Input: part model. Units: mm. Frame: model coordinates. A direction names the side the tool comes from. Give positions to 0.01 mm unless a question says otherwise; leave off trailing zeros. Loops run counter-clockwise (first coordinate to the right, second up) from the corner with the lowest first, then second, coordinate; pieces in that order, holes last. Notation, with made-up numbers: M -27.75,-0.75 L 18.25,-0.75 A31 cw 18.25,36.25 Z; hole C 72.5,-33.75 d11. An arc over 180 degrees is marked long. Answer as a JSON object with one key per item and string values. Group by question number.
1) First-contact query: P1, Ø1.5, axis at y = 18, z = 618, coming from the -X side; P2, Ø6, axis at x = 7, y = 14.5, coming from the +Z side. Flat tips, straight axial feed; report the tip coordinate or a pass-through.
2) Ray query, L1, parallel to X at y = 7.75, z = 55.5 (3 decimals); L2, parallel to Y at x = 0.8, z = 12.7. Return the intervals inside material, ascending.
3) Access query for faces 1 (the flat face through (24, 13, 0)), 2 (the flat face through (13, 22.225, 376)). Directions: +Z, -Z, +X, -X, +Y, -Y. A direction counts if a zero-diameter tool reaches every point of the face in a straight line with its end or side. Return the directions, or none.
4) Section query C-C on y = 12.7. Return loops of the section in (x, z) (3 decimals).
5) Section query A-A on z = 12.7. Return loops of the section in (x, y) (3 decimals), plus the area to 3 significant figures.
6) Draft query along Y for faces 3 (the cylindrical face through (23.79, 16.99, 8.02)), 4 (the flat face through (13, 25.4, 376)), 5 (the flat face through (0, 13, 376)). Return one class per face: +Y half, -Y half, draft (parallel to the pull), parting line (faces both ways), or undercut.
7) Section query B-B on x = 10.5. Return loops of the section in (y, z) (3 decimals).
8) Section query D-D on z = 453.5. Return loops of the section in (x, y) (3 decimals).
Autodesk Inventor part; units mm, degrees
ref_plane "YZ Plane" through (0, 0, 0) normal (1, 0, 0) x (0, 1, 0)
ref_plane "XZ Plane" through (0, 0, 0) normal (0, 1, 0) x (-1, 0, 0)
ref_plane "XY Plane" through (0, 0, 0) normal (0, 0, 1) x (1, 0, 0)
sketch "Sketch1" plane through (0, 0, 0) normal (0, 0, 1) x (1, 0, 0)
  line L0 (0, 0) -> (25.4, 0)
  line L1 (25.4, 0) -> (25.4, 25.4)
  line L2 (25.4, 25.4) -> (0, 25.4)
  line L3 (0, 25.4) -> (0, 0)
  line L4 (3.175, 3.175) -> (22.225, 3.175)
  line L5 (22.225, 3.175) -> (22.225, 22.225)
  line L6 (22.225, 22.225) -> (3.175, 22.225)
  line L7 (3.175, 22.225) -> (3.175, 3.175)
  dimension "d0" = 25.4
  dimension "d1" = 25.4
  dimension "d2" = 3.175
extrude "Extrusion1" add sketch "Sketch1" along normal blind 762
sketch "Sketch2" plane through (0, 0, 0) normal (-1, 0, 0) x (0, 0, 1)
  circle A0 centre (12.7, 12.7) radius 6.35
  line L0 (0, 25.4) -> (0, 0)
  line L1 (0, 0) -> (762, 0)
  dimension "d5" = 12.7
  dimension "d6" = 12.7
  dimension "d7" = 12.7
extrude "Extrusion2" cut sketch "Sketch2" against normal blind 25.4
properties part number "support bar" material "Aluminum 6061"
Output:
{
 "1": {"P1": "stops at x = 0", "P2": "passes through"},
 "2": {"L1": "x = 0 to 3.175, 22.225 to 25.4", "L2": "y = 0 to 6.35, 19.05 to 25.4"},
 "3": {"face 1": "-Z, +X, -X, +Y, -Y", "face 2": "+Z, -Z"},
 "4": {"outline": "M 0,0 L 3.175,0 L 3.175,6.35 L 0,6.35 Z; M 0,19.05 L 3.175,19.05 L 3.175,762 L 0,762 Z; M 22.225,0 L 25.4,0 L 25.4,6.35 L 22.225,6.35 Z; M 22.225,19.05 L 25.4,19.05 L 25.4,762 L 22.225,762 Z"},
 "5": {"outline": "M 0,0 L 25.4,0 L 25.4,6.35 L 22.225,6.35 L 22.225,3.175 L 3.175,3.175 L 3.175,6.35 L 0,6.35 Z; M 0,19.05 L 3.175,19.05 L 3.175,22.225 L 22.225,22.225 L 22.225,19.05 L 25.4,19.05 L 25.4,25.4 L 0,25.4 Z", "area": "202 mm^2"},
 "6": {"face 3": "undercut", "face 4": "+Y half", "face 5": "draft"},
 "7": {"outline": "M 0,0 L 3.175,0 L 3.175,762 L 0,762 Z; M 22.225,0 L 25.4,0 L 25.4,762 L 22.225,762 Z"},
 "8": {"outline": "M 0,0 L 25.4,0 L 25.4,25.4 L 0,25.4 Z; hole M 3.175,3.175 L 22.225,3.175 L 22.225,22.225 L 3.175,22.225 Z"}
}
